Design review of the part shown in the three views and the two pictorial views. Dimensions are in mm from the part's minimum x, y and z. Coordinates: 2 decimals unless noted, no trailing zeros. Loops run counter-clockwise (first coordinate to the right, second up) from the corner with the lowest first, then second, coordinate; pieces in that order, holes last.
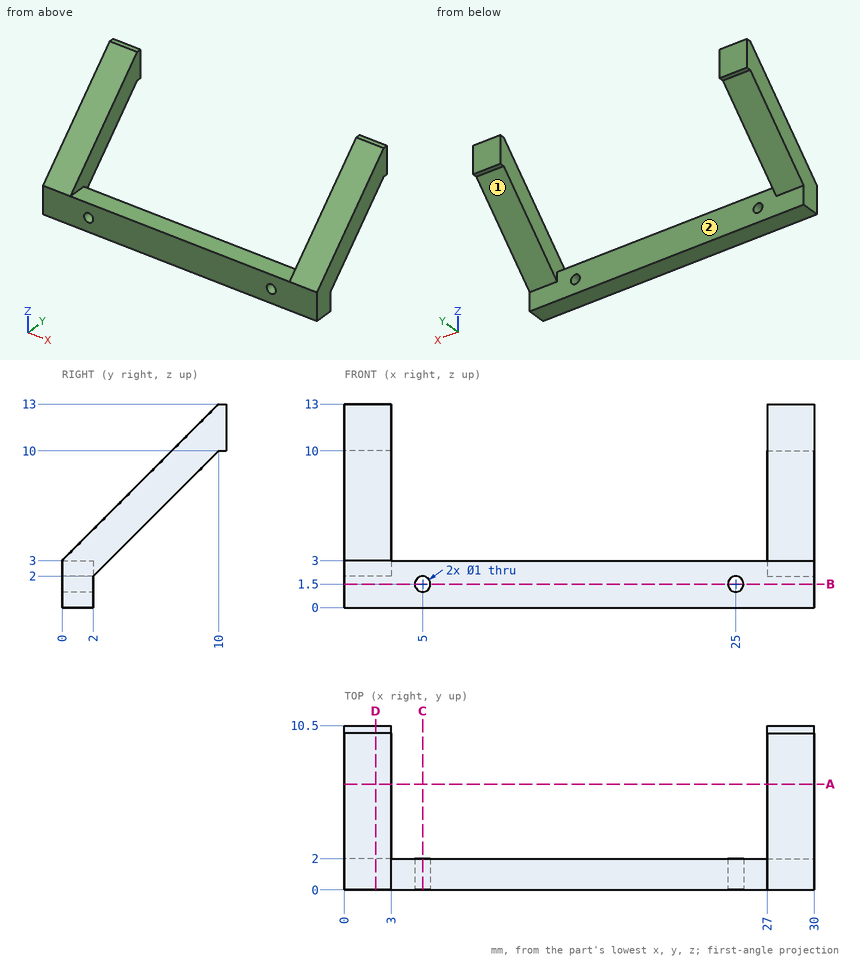
Q1. Consider section A-A (y = 6.75). State the section outline as (x, z) points.
Q2. Consider section B-B (z = 1.5). State the section outline as (x, y) points.
Q3. Wall thickness on probe 1 along X at (y, z) = (0.8, 1.5); probe 2 along X at (y, z) = (8, 10.75); probe 3 along Y at (x, z) = (27.5, 9.75): over which ranges is each line inside the solid? List them lowest first.
Q4. The part is to be moulded in two halves that separate along X. For the marked faces 1 and 2, say which applies: +X half, -X half, draft (parallel to the pull), parting line (faces both ways), or undercut.
Q5. For pin 1 Ø2.5 at (x, z) = (11, 2) entering from +Y; pin 2 Ø1 at (x, y) = (19.5, 1) entering from +Z; pin 3 Ø0.6 at (x, y) = (1.5, 10) entering from -Z, all flat-tipped, find the tip position at first contact; note any pin that passes through.
Q6. Consider section D-D (x = 2). State the section outline as (y, z) points.
Q7. Consider section C-C (x = 5). State the section outline as (y, z) points.
Model answer:
1. outline: (0, 6.75) - (3, 6.75) - (3, 9.75) - (0, 9.75) - close; (27, 6.75) - (30, 6.75) - (30, 9.75) - (27, 9.75) - close
2. outline: (0, 0) - (4.5, 0) - (4.5, 2) - (0, 2) - close; (5.5, 0) - (24.5, 0) - (24.5, 2) - (5.5, 2) - close; (25.5, 0) - (30, 0) - (30, 2) - (25.5, 2) - close
3. probe 1: x = 0 to 4.5, 5.5 to 24.5, 25.5 to 30
3. probe 2: x = 0 to 3, 27 to 30
3. probe 3: y = 6.75 to 9.75
4. face 1: draft
4. face 2: undercut
5. pin 1: stops at y = 2
5. pin 2: stops at z = 3
5. pin 3: stops at z = 9.7
6. outline: (0, 0) - (2, 0) - (2, 2) - (10, 10) - (10.5, 10) - (10.5, 13) - (10, 13) - (0, 3) - close
7. outline: (0, 0) - (2, 0) - (2, 1) - (0, 1) - close; (0, 2) - (2, 2) - (2, 3) - (0, 3) - close
